The listing builds one solid part. Answer for the finished solid, in the listing's coordinates (mm). A direction names the side the tool comes from. Round coordinates to 2 decimals unless told otherwise and drop trailing zeros. Order: outer loops, then holes, each group sorted by start corner. A loop starts at its lowest first (then second) coordinate and runs counter-clockwise, first axis right, second up. Notation, with made-up numbers: (72, 35) - (108, 35) arc R21 cw to (108, 44) - close; hole circle Ø5 at (19, 89.5). An arc over 180 degrees is marked (long way). Write item = value, one per line.
from build123d import *

# Parameters (mm, degrees)
F0_W     = 2.5
F0_H     = 55
F1_DEPTH = 35
F0_W_2   = 45
F2_DEPTH = 2.5
F4_D     = 13
F4_DEPTH = 12
F5_D     = 13
F5_DEPTH = 12


with BuildPart() as f1:
    # F0 (on Top) → F1 (new body)
    with BuildSketch(Plane.XY):
        Polygon((-47.320926, 2.681236), (-49.820926, 2.681236), (-49.820926, 0.181236), (0.179074, 0.181236), (0.179074, 2.681236), (-2.320926, 2.681236), align=None)
        with Locations((-48.570926, 30.181236)):
            Rectangle(F0_W, F0_H)
        Polygon((0.179074, 60.181236), (-49.820926, 60.181236), (-49.820926, 57.681236), (-47.320926, 57.681236), (-2.320926, 57.681236), (0.179074, 57.681236), align=None)
        with Locations((-1.070926, 30.181236)):
            Rectangle(F0_W, F0_H)
    extrude(amount=F1_DEPTH)

    # F0 (on Top) → F2 (join)
    with BuildSketch(Plane.XY):
        with Locations((-24.820926, 30.181236)):
            Rectangle(F0_W_2, F0_H)
    extrude(amount=F2_DEPTH)

    # F4
    with Locations(Plane(origin=(-49.820926, 0, 0), x_dir=(0, -1, 0), z_dir=(-1, 0, 0))):
        with Locations((-43.28923, 17.549016)):
            Hole(F4_D / 2, depth=F4_DEPTH)

    # F5
    with Locations(Plane(origin=(-49.820926, 0, 0), x_dir=(0, -1, 0), z_dir=(-1, 0, 0))):
        with Locations((-17.78923, 17.549016)):
            Hole(F5_D / 2, depth=F5_DEPTH)


solid = f1.part
Q1. Find the intervals of material crossed by line 1 (X direction, y = 55, z = 5); line 2 (Y direction, x = -2.5, z = 15); line 3 (Z direction, x = -15, y = 23), in increasing order. Write a range as from..to.
Model answer:
line_1 = -49.82..-47.32, -2.32..0.18
line_2 = 0.18..2.68, 57.68..60.18
line_3 = 0..2.5
Q2. Determine the mould class of faces 1 (the face through (-25, 0.181, 17)), 2 (the face through (-25, 31, 0)), 3 (the face through (-47.321, 30, 19)), 4 (the face through (-48.55, 49.49, 19.5)) for opening direction Y: released by +Y, released by -Y, zero draft, split by the parting line, or undercut.
Model answer:
face_1 = released by -Y
face_2 = zero draft
face_3 = undercut
face_4 = undercut
Q3. Section D-D on z = 28 is taken. Determine the outline of the cut face in (x, y).
Model answer:
outline = (-49.82, 0.18) - (0.18, 0.18) - (0.18, 60.18) - (-49.82, 60.18) - close; hole (-47.32, 2.68) - (-2.32, 2.68) - (-2.32, 57.68) - (-47.32, 57.68) - close
Q4. Flat-ended cylindrical pins translate along their axes: P1, Ø3, axis at x = -32.5, y = 53, coming from the -Z side; P2, Ø10.5, axis at y = 17.79, z = 17.55, coming from the -X side; P3, Ø22.5, axis at x = -26, y = 35.5, coming from the +Z side. Find the tip coordinate at first contact, or state that the pin passes through.
Model answer:
P1 = 0
P2 = -2.32
P3 = 2.5
Q5. Section B-B on y = 23 is taken. Determine the outline of the cut face in (x, z).
Model answer:
outline = (-49.82, 0) - (0.18, 0) - (0.18, 35) - (-2.32, 35) - (-2.32, 2.5) - (-47.32, 2.5) - (-47.32, 13.66) - (-49.82, 13.66) - close; (-49.82, 21.43) - (-47.32, 21.43) - (-47.32, 35) - (-49.82, 35) - close
Q6. Section C-C on x = -7 is taken. Determine the outline of the cut face in (y, z).
Model answer:
outline = (0.18, 0) - (60.18, 0) - (60.18, 35) - (57.68, 35) - (57.68, 2.5) - (2.68, 2.5) - (2.68, 35) - (0.18, 35) - close
Q7. For faces 5 (the face through (-25, 2.681, 19)), 6 (the face through (-49, 17, 24)), 7 (the face through (0.179, 30, 17)), determine the directions among +Z, -Z, +X, -X, +Y, -Y from which every point of the face is accessible in a straight line to the end or side of a thin tool.
Model answer:
face_5 = +Z
face_6 = -X
face_7 = +Z, -Z, +X, +Y, -Y
Q8. Section A-A on z = 22 is taken. Determine the outline of the cut face in (x, y), then the cut area to 3 significant figures.
Model answer:
outline = (-49.82, 0.18) - (0.18, 0.18) - (0.18, 60.18) - (-49.82, 60.18) - (-49.82, 48.03) - (-47.32, 48.03) - (-47.32, 57.68) - (-2.32, 57.68) - (-2.32, 2.68) - (-47.32, 2.68) - (-47.32, 13.05) - (-49.82, 13.05) - close; (-49.82, 22.53) - (-47.32, 22.53) - (-47.32, 38.55) - (-49.82, 38.55) - close
area = 478 mm^2
